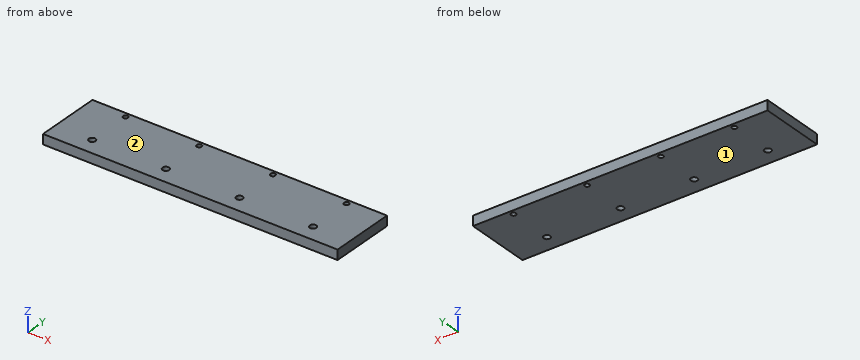
```python
from build123d import *

# Parameters (mm, degrees)
SKETCH1_W           = 360
SKETCH1_H           = 80
BOSS_EXTRUDE1_DEPTH = 12
CUT_EXTRUDE1_REACH  = 186.781
SKETCH2_R           = 3
SKETCH2_R_2         = 4
LPATTERN1_COUNT     = 4
LPATTERN1_PITCH     = 90


with BuildPart() as part:
    # Sketch1 → Boss-Extrude1 (new body)
    with BuildSketch(Plane.XY):
        Rectangle(SKETCH1_W, SKETCH1_H)
    extrude(amount=BOSS_EXTRUDE1_DEPTH)

    # Sketch2 → Cut-Extrude1 (cut, up to next)
    with BuildSketch(Plane.XY.offset(12), mode=Mode.PRIVATE) as cut_extrude1_sk1:
        with Locations((-135, 34)):
            Circle(SKETCH2_R)
    cut_extrude1_tool1 = extrude(cut_extrude1_sk1.sketch, amount=-CUT_EXTRUDE1_REACH, mode=Mode.PRIVATE) & part.part
    # Sketch2 → Cut-Extrude1 (cut, up to next)
    with BuildSketch(Plane.XY.offset(12), mode=Mode.PRIVATE) as cut_extrude1_sk2:
        with Locations((-135, -20)):
            Circle(SKETCH2_R_2)
    cut_extrude1_tool2 = extrude(cut_extrude1_sk2.sketch, amount=-CUT_EXTRUDE1_REACH, mode=Mode.PRIVATE) & part.part
    cut_extrude1_1 = cut_extrude1_tool1.solids().sort_by_distance((-135, 34, 12))[0]
    add(cut_extrude1_1, mode=Mode.SUBTRACT)
    cut_extrude1_2 = cut_extrude1_tool2.solids().sort_by_distance((-135, -20, 12))[0]
    add(cut_extrude1_2, mode=Mode.SUBTRACT)
    cut_extrude1 = cut_extrude1_1 + cut_extrude1_2  # Cut-Extrude1 as one shape, for the pattern or mirror that repeats it

    # LPattern1: Cut-Extrude1 ×4
    with Locations(*[(i * LPATTERN1_PITCH, 0, 0) for i in range(1, LPATTERN1_COUNT)]):
        add(cut_extrude1, mode=Mode.SUBTRACT)


solid = part.part
```
Input: part model. Units: mm. Frame: model coordinates. Face numbers are marked on the shaded views. Round coordinates to 2 decimals unless told otherwise and drop trailing zeros. Loops run counter-clockwise (first coordinate to the right, second up) from the corner with the lowest first, then second, coordinate; pieces in that order, holes last. Notation, with made-up numbers: (-2, -21.75) - (51, -21.75) arc R35 ccw to (51, 12.25) - close; hole circle Ø3 at (33, 63). An arc over 180 degrees is marked (long way). One line per item, written item: value. Start each with the question number.
(1) Section B-B, the plane x = -135. Return loops of the section in (y, z).
(2) Contact query for a flat-ended pin moving along its axis: P1, Ø13, axis at x = -45, y = -20, coming from the +Z side. Output: stop coordinate, or through.
(3) Draft query along Z for the marked faces 1 and 2. Return one class per face: +Z half, -Z half, draft (parallel to the pull), parting line (faces both ways), or undercut.
(4) Ray query, line 1 (Y direction, x = -45, z = 3). Return the intervals inside material, ascending. Write a range as [from, to].
(5) Section A-A, the plane y = 34. Return loops of the section in (x, z), plus the area to 3 significant figures.
Results below:
1. outline: (-40, 0) - (-24, 0) - (-24, 12) - (-40, 12) - close; (-16, 0) - (31, 0) - (31, 12) - (-16, 12) - close; (37, 0) - (40, 0) - (40, 12) - (37, 12) - close
2. P1: z = 12
3. face 1: -Z half
3. face 2: +Z half
4. line 1: [-40, -24], [-16, 31], [37, 40]
5. outline: (-180, 0) - (-138, 0) - (-138, 12) - (-180, 12) - close; (-132, 0) - (-48, 0) - (-48, 12) - (-132, 12) - close; (-42, 0) - (42, 0) - (42, 12) - (-42, 12) - close; (48, 0) - (132, 0) - (132, 12) - (48, 12) - close; (138, 0) - (180, 0) - (180, 12) - (138, 12) - close
5. area: 4,030 mm^2
